Model file for the job. Use its own axes, mm. A direction names the side the tool comes from. Round coordinates to 2 decimals unless told otherwise and drop trailing zeros. Order: outer loops, then holes, each group sorted by start corner. A loop starts at its lowest first (then second) coordinate and runs counter-clockwise, first axis right, second up. Notation, with made-up numbers: (72, -15.5) - (125, -15.5) arc R25 cw to (125, -2.5) - close; hole circle Ø3 at (-17, 24). An arc over 180 degrees is marked (long way). Write item = value, one per line. Start each with the question number.
from build123d import *

# Parameters (mm, degrees)
F0_R        = 19
F1_DEPTH    = 3.42
F2_T1_DEPTH = 28.42
F2_T3_DEPTH = 28.2950568544
F4_D        = 6.5
F5_D        = 5.5
F6_D        = 8.5
F7_D        = 7.14
F8_R        = 4.5
F9_DEPTH    = 5.5
F10_D       = 4.1
F10_DEPTH   = 2.081


# Not quite as in the source:
# - a fillet or chamfer that OpenCascade refuses, or shapes differently, is made with other operations: its cross-section is extruded or revolved along the edge and cut away or added
# - a feature names something its author has since deleted; it is built from what else it names


with BuildPart() as f1:
    # F0 (on Front) → F1 (new body)
    with BuildSketch(Plane.XZ):
        with BuildLine():
            Line((-80, -107.5), (80, -107.5))
            Line((80, -107.5), (80, 107.5))
            Line((80, 107.5), (3.175, 107.5))
            Line((3.175, 107.5), (3.175, 102.999261314))
            ThreePointArc((3.175, 102.999261314), (0, 91.15), (-3.175, 102.999261314))
            Line((-3.175, 102.999261314), (-3.175, 107.5))
            Line((-3.175, 107.5), (-80, 107.5))
            Line((-80, 107.5), (-80, -107.5))
        make_face()
        with Locations((34.285, 52.5)):
            Circle(F0_R, mode=Mode.SUBTRACT)
    extrude(amount=F1_DEPTH)

    # F2: fillet of radius 5 on 6 edges, made by hand

    # F2_s2 → F2_t1 (cut)
    with BuildSketch(Plane.XZ.offset(-12.5)):
        with BuildLine():
            ThreePointArc((-75, 107.5), (-78.5355339059, 106.0355339059), (-80, 102.5))
            Line((-80, 102.5), (-80, 107.5))
            Line((-80, 107.5), (-75, 107.5))
        make_face()
        with BuildLine():
            ThreePointArc((75, -107.5), (78.5355339059, -106.0355339059), (80, -102.5))
            Line((80, -102.5), (80, -107.5))
            Line((80, -107.5), (75, -107.5))
        make_face()
        with BuildLine():
            ThreePointArc((-80, -102.5), (-78.5355339059, -106.0355339059), (-75, -107.5))
            Line((-75, -107.5), (-80, -107.5))
            Line((-80, -107.5), (-80, -102.5))
        make_face()
        with BuildLine():
            ThreePointArc((80, 102.5), (78.5355339059, 106.0355339059), (75, 107.5))
            Line((75, 107.5), (80, 107.5))
            Line((80, 107.5), (80, 102.5))
        make_face()
    extrude(amount=F2_T1_DEPTH, mode=Mode.SUBTRACT)

    # F2_s4 → F2_t3 (cut)
    with BuildSketch(Plane.XZ.offset(-12.4375284272)):
        with BuildLine():
            ThreePointArc((-8.1500113709, 107.5), (-4.7956341239, 106.2078502242), (-3.175, 102.999261314))
            Line((-3.175, 102.999261314), (-3.175, 107.5))
            Line((-3.175, 107.5), (-8.1500113709, 107.5))
        make_face()
        with BuildLine():
            ThreePointArc((8.1500113709, 107.5), (4.7956341239, 106.2078502242), (3.175, 102.999261314))
            Line((3.175, 102.999261314), (3.175, 107.5))
            Line((3.175, 107.5), (8.1500113709, 107.5))
        make_face()
    extrude(amount=F2_T3_DEPTH, mode=Mode.SUBTRACT)

    # F4 (through all)
    with Locations(Plane.XZ.offset(3.42)):
        with Locations((-42, 79.5), (-10, 79.5), (-42, 14.5), (-10, 14.5)):
            Hole(F4_D / 2)

    # F5 (through all)
    with Locations(Plane.XZ.offset(3.42)):
        with Locations((-72, 47.5), (-72, 27.5), (72, 47.5), (72, 27.5), (-57.5, 97.5), (-26.5, 97.5), (-67, 12.5), (67, 12.5), (-42, 97.5)):
            Hole(F5_D / 2)

    # F6 (through all)
    with Locations(Plane.XZ.offset(3.42)):
        with Locations((10.5, 12.5), (40.5, 12.5)):
            Hole(F6_D / 2)

    # F7 (through all)
    with Locations(Plane.XZ.offset(3.42)):
        with Locations((-67, -94.5), (67, -94.5)):
            Hole(F7_D / 2)

    # F8 (on face) → F9 (join)
    with BuildSketch(Plane.XZ.offset(3.42)):
        with Locations((10.5, 76.07)):
            Circle(F8_R)
        with Locations((58.07, 76.07)):
            Circle(F8_R)
        with Locations((58.07, 28.93)):
            Circle(F8_R)
        with Locations((10.5, 28.93)):
            Circle(F8_R)
    extrude(amount=-F9_DEPTH)

    # F10 (through all, one way)
    with BuildSketch(Plane.XZ):
        with Locations((10.5, 76.07), (58.07, 76.07), (10.5, 28.93), (58.07, 28.93)):
            Circle(F10_D / 2)
    extrude(amount=-F10_DEPTH, mode=Mode.SUBTRACT)


solid = f1.part
Item 1: Which spindle directions (+Z, -Z, +X, -X, +Y, -Y) get a long thin tool onto all of the face, cutting with end or side? Do faces 4 (the face through (8.873, 1.025, 27.683)), 5 (the face through (-78.57, -1.69, -106)), 6 (the face through (-4.83, -1.69, 106.24)). Say none if no direction does.
Item 2: Mould opens along Z. For faces 1 (the face through (78.5, -1.69, -106.07)), 2 (the face through (8, 2.08, 29)), 3 (the face through (43.052, -1.686, 35.644)) say: +Z half, -Z half, draft (parallel to the pull), parting line (faces both ways), or undercut.
Item 3: Drop flat-ended pins along their axis: pin 1 (1 mm diameter, centred on x = -4.5, y = 1, fed in from -Z); pin 2 (7 mm diameter, centred on x = 72, z = 27.5, fed in from -Y); pin 3 (1.2 mm diameter, centred on x = 11, z = 76, fed in from +Y). Give the stop position or say it passes through.
Item 4: Saw through at D-D, the plane z = -31. Give the cut face in (x, y), then the cut area to 3 significant figures.
Item 5: Saw through at C-C, the plane x = 40.5. Give the cut face in (y, z), then the cut area to 3 significant figures.
Item 6: Probe L1, parallel to Z at x = -72, y = -0.95; L2, parallel to Z at x = -10, y = -2.4; L3, parallel to Z at x = 10.5, y = 1.65. List the from-to ranges inside material, lowest first.
Item 7: Saw through at B-B, the plane x = -42. Give the cut face in (y, z).
Item 8: Saw through at A-A, the plane y = -2.05. Give the number of separate pieces and of enclosed holes in the cut face, then the cut area to 3 significant figures.
Check sheet entries:
q1.face_4 = +Y
q1.face_5 = -Z, -X, +Y, -Y
q1.face_6 = +Z, +Y, -Y
q2.face_1 = -Z half
q2.face_2 = draft
q2.face_3 = undercut
q3.pin_1 = through
q3.pin_2 = -3.42
q3.pin_3 = 0
q4.outline = (-80, -3.42) - (80, -3.42) - (80, 0) - (-80, 0) - close
q4.area = 547 mm2
q5.outline = (-3.42, -107.5) - (0, -107.5) - (0, 8.25) - (-3.42, 8.25) - close; (-3.42, 16.75) - (0, 16.75) - (0, 34.55) - (-3.42, 34.55) - close; (-3.42, 70.45) - (0, 70.45) - (0, 107.5) - (-3.42, 107.5) - close
q5.area = 583 mm2
q6.L1 = -107.5 to 24.75, 30.25 to 44.75, 50.25 to 107.5
q6.L2 = -107.5 to 11.25, 17.75 to 76.25, 82.75 to 107.5
q6.L3 = 24.43 to 26.88, 30.98 to 33.43, 71.57 to 74.02, 78.12 to 80.57
q7.outline = (-3.42, -107.5) - (0, -107.5) - (0, 11.25) - (-3.42, 11.25) - close; (-3.42, 17.75) - (0, 17.75) - (0, 76.25) - (-3.42, 76.25) - close; (-3.42, 82.75) - (0, 82.75) - (0, 94.75) - (-3.42, 94.75) - close; (-3.42, 100.25) - (0, 100.25) - (0, 107.5) - (-3.42, 107.5) - close
q8.separate_pieces = 1
q8.enclosed_holes = 18
q8.area = 32,500 mm2
